Model file for the job. Use its own axes, mm. A direction names the side the tool comes from. Round coordinates to 2 decimals unless told otherwise and drop trailing zeros. Order: outer loops, then holes, each group sorted by start corner. A loop starts at its lowest first (then second) coordinate and runs counter-clockwise, first axis right, second up. Notation, with made-up numbers: M -3,8.25 L 3,8.25 A35 cw 3,40.25 Z; hole C 77,-4 d11. An arc over 180 degrees is marked long. Return JSON: item names as keys, results as strings. Group by question number.
Item 1: Slice it at B-B on y = -16. Write the cut outline in (x, z), then the cut area to 3 significant figures.
Item 2: Slice it at D-D on y = -8. Write the cut outline in (x, z).
Item 3: Probe line 1 along Y through (x, z) = (-7.95, 0); line 2 along Y through (x, z) = (-0.75, 5.25); line 3 along X through (y, z) = (-14.5, -6.5). List the from-to ranges inside material, lowest first.
Item 4: Pin check, flat tips, straight feed: pin 1 Ø1 at (y, z) = (-6.5, -8) entering from -X; pin 2 Ø8 at (x, y) = (7.5, -2) entering from +Z; pin 3 Ø5 at (x, y) = (7.5, -4.5) entering from -Z. Stop position of each tip, or through.
Item 5: Slice it at A-A on y = -10. Write the cut outline in (x, z), then the cut area to 3 significant figures.
Item 6: Pull direction Z, two halves, no side cores. Call faces 4 (the face through (9, -2.5, -5)), 5 (the face through (-8.349, -5.615, 0.751)), 6 (the face through (0, -10, -9)), 7 (the face through (-0.44, -4.75, -9.99)): pulls with the +Z half, pulls with the -Z half, needs draft (parallel to the pull), parting line crosses it, or undercut.
Item 7: Which spindle directions (+Z, -Z, +X, -X, +Y, -Y) get a long thin tool onto all of the face, cutting with end or side? Do faces 1 (the face through (-6.25, -10, 2)), 2 (the face through (3.2, -11.7, 10)), 3 (the face through (-0.44, -1.75, -9.99)). Say none if no direction does.
Item 8: Slice it at C-C on z = 0. Give the number of separate pieces and of enclosed holes in the cut face, then the cut area to 3 significant figures.
from build123d import *

# Parameters (mm, degrees)
SKETCH2_R               = 10.5
BOSS_EXTRUDE1_DEPTH     = 18.5
CUT_EXTRUDE1_DEPTH      = 16.5
SKETCH4_R               = 2.5
CUT_EXTRUDE2_DEPTH      = 11.5
CUT_EXTRUDE2_DEPTH_BACK = 11.5
SKETCH5_W               = 0.5
SKETCH5_H               = 0.5
LPATTERN1_COUNT         = 5
LPATTERN1_PITCH         = 1


with BuildPart() as part:
    # Sketch2 → Boss-Extrude1 (new body)
    with BuildSketch(Plane(origin=(0, 0, 0), x_dir=(1, 0, 0), z_dir=(0, 1, 0))):
        with Locations(Location((0, 0, 0), (0, 0, 270))):  # turned: the seam where the file's is
            Circle(SKETCH2_R)
    extrude(amount=-BOSS_EXTRUDE1_DEPTH)

    # Sketch3 → Cut-Extrude1 (cut)
    with BuildSketch(Plane.XZ.offset(18.5)):
        with BuildLine():
            Line((-6.25, 6.475916923), (-6.25, -6.475916923))
            ThreePointArc((-6.25, -6.475916923), (0, -9), (6.25, -6.475916923))
            Line((6.25, -6.475916923), (6.25, 6.475916923))
            ThreePointArc((6.25, 6.475916923), (0, 9), (-6.25, 6.475916923))
        make_face()
    extrude(amount=-CUT_EXTRUDE1_DEPTH, mode=Mode.SUBTRACT)

    # Sketch4 → Cut-Extrude2 (cut, two sides)
    with BuildSketch(Plane(origin=(0, 0, 0), x_dir=(0, 0, -1), z_dir=(1, 0, 0))) as cut_extrude2_sk:
        with Locations(Location((0, -8, 0), (0, 0, 90))):  # turned: the seam where the file's is
            Circle(SKETCH4_R)
    extrude(amount=CUT_EXTRUDE2_DEPTH, mode=Mode.SUBTRACT)
    extrude(cut_extrude2_sk.sketch, amount=-CUT_EXTRUDE2_DEPTH_BACK, mode=Mode.SUBTRACT)

    # Sketch5 → Cut-Revolve1 (revolve, cut)
    with BuildSketch(Plane(origin=(0, 0, 0), x_dir=(0, 0, -1), z_dir=(1, 0, 0)), mode=Mode.PRIVATE) as cut_revolve1_sk:
        with Locations((10.25, -0.75)):
            Rectangle(SKETCH5_W, SKETCH5_H)
    cut_revolve1 = revolve(cut_revolve1_sk.sketch.rotate(Axis((0, 0, 0), (0, -1, 0)), 180), axis=Axis((0, 0, 0), (0, -1, 0)), mode=Mode.SUBTRACT)  # turned: the seam where the file's is

    # LPattern1: Cut-Revolve1 ×5
    with Locations(*[(0, -i * LPATTERN1_PITCH, 0) for i in range(1, LPATTERN1_COUNT)]):
        add(cut_revolve1, mode=Mode.SUBTRACT)


solid = part.part
Output values:
{
 "1": {"outline": "C 0,0 d21; hole M -6.25,-6.48 A9 ccw 6.25,-6.48 L 6.25,6.48 A9 ccw -6.25,6.48 Z", "area": "141 mm²"},
 "2": {"outline": "M -10.2,-2.5 A10.5 ccw 10.2,-2.5 L 6.25,-2.5 L 6.25,-6.48 A9 cw -6.25,-6.48 L -6.25,-2.5 Z; M -10.2,2.5 L -6.25,2.5 L -6.25,6.48 A9 cw 6.25,6.48 L 6.25,2.5 L 10.2,2.5 A10.5 ccw Z"},
 "3": {"line 1": "-18.5 to -10.5, -5.5 to 0", "line 2": "-2 to 0", "line 3": "-8.25 to -6.22, 6.22 to 8.25"},
 "4": {"pin 1": "x = -7.35", "pin 2": "z = 9.9", "pin 3": "z = -9.23"},
 "5": {"outline": "M -10.39,-1.5 A10.5 ccw 10.39,-1.5 L 6.25,-1.5 L 6.25,-6.48 A9 cw -6.25,-6.48 L -6.25,-1.5 Z; M -10.39,1.5 L -6.25,1.5 L -6.25,6.48 A9 cw 6.25,6.48 L 6.25,1.5 L 10.39,1.5 A10.5 ccw Z", "area": "116 mm²"},
 "6": {"face 4": "needs draft", "face 5": "undercut", "face 6": "undercut", "face 7": "parting line crosses it"},
 "7": {"face 1": "-Y", "face 2": "+Y, -Y", "face 3": "none"},
 "8": {"separate pieces": "3", "enclosed holes": "0", "area": "137 mm²"}
}
